Autodesk Inventor part; units mm, degrees
ref_plane "YZ Plane" through (0, 0, 0) normal (1, 0, 0) x (0, 1, 0)
ref_plane "XZ Plane" through (0, 0, 0) normal (0, 1, 0) x (-1, 0, 0)
ref_plane "XY Plane" through (0, 0, 0) normal (0, 0, 1) x (1, 0, 0)
sketch "Sketch1" plane through (0, 0, 0) normal (0, 0, 1) x (1, 0, 0)
  line L0 (0, 0) -> (20, 0)
  line L1 (20, 0) -> (20, 34)
  line L2 (20, 34) -> (0, 34)
  line L3 (0, 34) -> (0, 0)
  dimension "d0" = 20
  dimension "d1" = 34
extrude "Extrusion1" add sketch "Sketch1" along normal blind 9.5
sketch "Sketch2" plane through (20, 0, 0) normal (1, 0, 0) x (0, 0, -1)
  line L0 (0, 0) -> (0, 34)
  circle A0 centre (0.5, 18.5) radius 4
  dimension "d4" = 8
  dimension "d11" = 0.5
  dimension "d26" = 18.5
extrude "Extrusion2" cut sketch "Sketch2" against normal up to next
sketch "Sketch3" plane through (0, 0, 9.5) normal (-1, 0, 0) x (0, 0, 1)
  line L0 (-9.5, 14.5314) -> (-9.5, 0)
  line L1 (-9.5, 34) -> (-9.5, 22.4686)
  circle A0 centre (-10, 6.5) radius 4.4
  circle A1 centre (-10, 28.5) radius 4.4
  arc A2 (-9.5, 14.5314) -> (-9.5, 22.4686) centre (-10, 18.5) ccw
  dimension "d7" = 8.8
  dimension "d8" = 8.8
  dimension "d9" = 0.5
  dimension "d10" = 0.5
  dimension "d64" = 10
  dimension "d65" = 12
extrude "Extrusion3" cut sketch "Sketch3" against normal blind 7
sketch "Sketch7" plane through (20, 0, 9.5) normal (1, 0, 0) x (0, 0, -1)
  line L0 (9.5, 22.4686) -> (9.5, 34)
  circle A0 centre (9.5, 28.5) radius 2.5
  line L1 (9.5, 2.1285) -> (9.5, 14.5314)
  circle A1 centre (9.5, 6.5) radius 2.5
  arc A2 (9.5, 22.4686) -> (9.5, 14.5314) centre (10, 18.5) ccw
  dimension "d33" = 5
  dimension "d34" = 5
  dimension "d61" = 10
  dimension "d62" = 12
extrude "Extrusion7" add sketch "Sketch7" against normal up to surface (13 mm away)
sketch "Sketch8" plane through (0, 0, 9.5) normal (0, 0, 1) x (1, 0, 0)
  line L0 (20, 34) -> (0, 34)
  line L1 (0, 34) -> (0, 0)
  circle A0 centre (14, 28.5) radius 2
  circle A1 centre (14, 6.5314) radius 2
  line L2 (20, 22.4686) -> (20, 14.5314)
  line L3 (20, 22.4686) -> (0, 22.4686)
  line L4 (20, 14.5314) -> (20, 22.4686)
  line L5 (0, 14.5314) -> (20, 14.5314)
  line L6 (0, 22.4686) -> (0, 14.5314)
  dimension "d39" = 4
  dimension "d40" = 4
  dimension "d42" = 5.5
  dimension "d43" = 14
  dimension "d66" = 8
extrude "Extrusion8" cut sketch "Sketch8" against normal up to next contours A0 | A1
sketch "Sketch9" plane through (0, 34, 0) normal (0, 1, 0) x (1, 0, 0)
  line L0 (20, 0) -> (0, 0)
  line L1 (20, 0) -> (20, -9.5)
  circle A0 centre (10, 0) radius 1.6
  dimension "d48" = 3.2
  dimension "d49" = 10
extrude "Extrusion9" add sketch "Sketch9" against normal blind 6
sketch "Sketch10" plane through (0, 0, 9.5) normal (0, 0, 1) x (1, 0, 0)
  circle A0 centre (14, 28.5) radius 2
  circle A1 centre (14, 6.5314) radius 2
  circle A2 centre (14, 28.5) radius 3.5
  circle A3 centre (14, 6.5314) radius 3.5
  dimension "d52" = 7
  dimension "d53" = 7
extrude "Extrusion10" cut sketch "Sketch10" against normal blind 4
sketch "Sketch11" plane through (0, 0, 0) normal (0, -1, 0) x (1, 0, 0)
  line L0 (0, 0) -> (20, 0)
  line L1 (0, 0) -> (0, 9.5)
  circle A0 centre (10, -0.5) radius 5.5
  dimension "d56" = 11
  dimension "d57" = 10
  dimension "d58" = 0.5
extrude "Extrusion11" cut sketch "Sketch11" against normal blind 1
properties part number "YAxisIdlerCap" material "ABS Plastic"
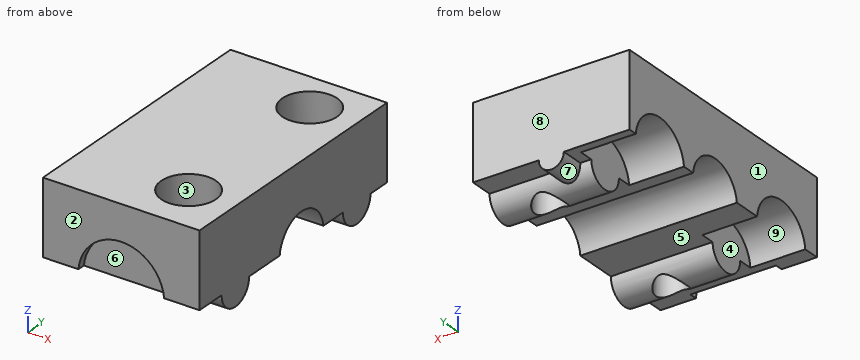
Could you check a few things on this model? Use its own coordinates, in mm. Face numbers are marked on the shaded views. A direction names the side the tool comes from. Give positions to 0.01 mm unless a question says otherwise; leave off trailing zeros. Order: outer loops, then holes, each group sorted by start corner. A loop starts at its lowest first (then second) coordinate and runs counter-clockwise, first axis right, second up. Notation, with made-up numbers: (-0.5, 50) -> (28.5, 50) arc R10 cw to (28.5, 57) -> close; hole circle Ø1 at (72.5, 9.25). An arc over 180 degrees is marked (long way). Return JSON: item names as keys, results as strings.
1. Thinking about a two-plate mould opening in Y: for the marked faces 6, 7, 8 and 9, which applies, pulls with the +Y half, pulls with the -Y half, needs draft (parallel to the pull), parting line crosses it, or undercut?
Answer list:
{"face 6": "pulls with the -Y half", "face 7": "needs draft", "face 8": "pulls with the +Y half", "face 9": "undercut"}
2. Imagine slicing it at B-B on x = 18.25. List the corners of the cut face in (y, z) for me.
Answer list:
{"outline": "(0, 0) -> (4, 0) arc R2.5 ccw to (9, 0) -> (14.53, 0) arc R4 cw to (22.47, 0) -> (26, 0) arc R2.5 ccw to (31, 0) -> (34, 0) -> (34, 9.5) -> (0, 9.5) -> close"}
3. Imagine slicing it at D-D on x = 14. List the corners of the cut face in (y, z) for me.
Answer list:
{"outline": "(0, 3.27) -> (1, 3.27) -> (1, 0) -> (4, 0) arc R2.5 ccw to (4.53, -1.54) -> (4.53, 5.5) -> (3.03, 5.5) -> (3.03, 9.5) -> (0, 9.5) -> close; (8.53, -1.46) arc R2.5 ccw to (9, 0) -> (14.53, 0) arc R4 cw to (22.47, 0) -> (26, 0) arc R2.5 ccw to (26.5, -1.5) -> (26.5, 5.5) -> (25, 5.5) -> (25, 9.5) -> (10.03, 9.5) -> (10.03, 5.5) -> (8.53, 5.5) -> close; (30.5, -1.5) arc R2.5 ccw to (31, 0) -> (34, 0) -> (34, 9.5) -> (32, 9.5) -> (32, 5.5) -> (30.5, 5.5) -> close"}
4. I need wall thicknesses on line 1 (Y direction, x = 6, z = 2); line 2 (Y direction, x = 12.5, z = -1); line 3 (Z direction, x = 8.75, y = 25). Which ranges of each line are inside material? Lowest first, please. Write a range as from..to.
Answer list:
{"line 1": "y = 1..2.88, 10.12..15.38, 21.62..24.88, 32.12..34", "line 2": "y = 4.21..5.21, 7.85..8.79, 26.21..27.18, 29.82..30.79", "line 3": "z = 0..9.5"}
5. For pin 1 Ø6.5 at (x, y) = (14, 28.5) entering from +Z; pin 2 Ø0.9 at (x, y) = (4.5, 32) entering from -Z; pin 3 Ø1.9 at (y, z) = (30, 1) entering from -X, each with a flat end and sliding along its axis, tell me the tip position at first contact or that it passes through.
Answer list:
{"pin 1": "stops at z = 5.5", "pin 2": "stops at z = 1.44", "pin 3": "stops at x = 7"}
6. Imagine slicing it at C-C on z = -0.5. List the corners of the cut face in (x, y) for me.
Answer list:
{"outline": "(7, 4.05) -> (20, 4.05) -> (20, 8.95) -> (7, 8.95) -> close; (7, 26.05) -> (20, 26.05) -> (20, 30.95) -> (11.52, 30.95) -> (11.52, 34) -> (8.48, 34) -> (8.48, 30.95) -> (7, 30.95) -> close; hole circle Ø4 at (14, 6.53); hole circle Ø4 at (14, 28.5)"}
7. Imagine slicing it at A-A on y = 28.5. List the corners of the cut face in (x, z) for me.
Answer list:
{"outline": "(0, 3.9) -> (7, 3.9) -> (7, -2.5) -> (12, -2.5) -> (12, 5.5) -> (10.5, 5.5) -> (10.5, 9.5) -> (0, 9.5) -> close; (16, -2.5) -> (20, -2.5) -> (20, 9.5) -> (17.5, 9.5) -> (17.5, 5.5) -> (16, 5.5) -> close"}
8. On a 3-axis mill with a long thin cutter (end or side, diameter ignored), from which of +Z, -Z, +X, -X, +Y, -Y can I reach the whole of each face in a straight line? I mean the marked faces 1, 2, 3, 4 and 5. Say none if no direction works.
Answer list:
{"face 1": "+Z, -Z, -X, +Y, -Y", "face 2": "+Z, -Z, +X, -X, -Y", "face 3": "+Z", "face 4": "-Z, -X", "face 5": "-Z, +X, -X"}
